CAD build for the part. Positions are in the model's coordinates, mm. A direction names the side the tool comes from. Give positions to 0.01 mm unless a question says otherwise; leave off trailing zeros. Write each loop counter-clockwise with the first axis right and the second up, starting at its lowest first coordinate (ties: lowest second). Pieces come first, ordered by that corner, then holes. Notation, with made-up numbers: (88.5, -23.75) -> (119.5, -23.75) arc R31 cw to (119.5, 13.25) -> close; hole circle Ø11 at (-16, -12). An arc over 180 degrees is marked (long way). Answer as a JSON object with one key per item and string values.
```python
from build123d import *

# Parameters (mm, degrees)
F0_R     = 9.525
F0_R_2   = 12.7
F1_DEPTH = 19.05
F2_R     = 34.925
F2_R_2   = 12.7
F3_DEPTH = 19.05
F4_R     = 34.925
F4_R_2   = 25.4
F5_DEPTH = 12.7
F7_DEPTH = 12.7


with BuildPart() as f1:
    # F0 (on Front) → F1 (new body)
    with BuildSketch(Plane.XZ):
        with BuildLine():
            Line((-60.325, -16.497784), (-22.225, -38.494829))
            ThreePointArc((-22.225, -38.494829), (-0.877898, -44.44133), (20.687394, -39.342524))
            Line((20.687394, -39.342524), (60.483871, -18.416429))
            ThreePointArc((60.483871, -18.416429), (71.607263, 0), (60.483871, 18.416429))
            Line((60.483871, 18.416429), (20.687394, 39.342524))
            ThreePointArc((20.687394, 39.342524), (-0.877898, 44.44133), (-22.225, 38.494829))
            Line((-22.225, 38.494829), (-60.325, 16.497784))
            ThreePointArc((-60.325, 16.497784), (-69.85, 0), (-60.325, -16.497784))
        make_face()
        with Locations((-50.8, 0)):
            Circle(F0_R, mode=Mode.SUBTRACT)
        Circle(F0_R_2, mode=Mode.SUBTRACT)
        with Locations((50.8, 0)):
            Circle(F0_R, mode=Mode.SUBTRACT)
    extrude(amount=F1_DEPTH)

    # F2 (on face) → F3 (join)
    with BuildSketch(Plane.XZ.offset(19.05)):
        Circle(F2_R)
        Circle(F2_R_2, mode=Mode.SUBTRACT)
    extrude(amount=F3_DEPTH)

    # F4 (on face) → F5 (join)
    with BuildSketch(Plane.XZ.offset(38.1)):
        Circle(F4_R)
        Circle(F4_R_2, mode=Mode.SUBTRACT)
    extrude(amount=F5_DEPTH)

    # F6 (on face) → F7 (cut)
    with BuildSketch(Plane.XZ.offset(50.8)):
        with BuildLine():
            Line((-6.35, 34.342876), (-6.35, 24.593444))
            ThreePointArc((-6.35, 24.593444), (0, 25.4), (6.35, 24.593444))
            Line((6.35, 24.593444), (6.35, 34.342876))
            ThreePointArc((6.35, 34.342876), (0, 34.925), (-6.35, 34.342876))
        make_face()
        with BuildLine():
            Line((34.342876, 6.35), (24.593444, 6.35))
            ThreePointArc((24.593444, 6.35), (25.4, 0), (24.593444, -6.35))
            Line((24.593444, -6.35), (34.342876, -6.35))
            ThreePointArc((34.342876, -6.35), (34.925, 0), (34.342876, 6.35))
        make_face()
        with BuildLine():
            Line((6.35, -34.342876), (6.35, -24.593444))
            ThreePointArc((6.35, -24.593444), (0, -25.4), (-6.35, -24.593444))
            Line((-6.35, -24.593444), (-6.35, -34.342876))
            ThreePointArc((-6.35, -34.342876), (0, -34.925), (6.35, -34.342876))
        make_face()
        with BuildLine():
            Line((-34.342876, -6.35), (-24.593444, -6.35))
            ThreePointArc((-24.593444, -6.35), (-25.4, 0), (-24.593444, 6.35))
            Line((-24.593444, 6.35), (-34.342876, 6.35))
            ThreePointArc((-34.342876, 6.35), (-34.925, 0), (-34.342876, -6.35))
        make_face()
    extrude(amount=-F7_DEPTH, mode=Mode.SUBTRACT)


solid = f1.part
```
1) Mould opens along X. For faces 6 (the flat face through (30, -45, 6.35)), 7 (the cylindrical face through (71.605, -9.392, -0.317)), 8 (the flat face through (-6.35, -45, -29)) say: released by +X, released by -X, zero draft, split by the parting line, or undercut.
Model answer:
{"face 6": "zero draft", "face 7": "released by +X", "face 8": "undercut"}
2) Slice it at B-B (z = 0). List the corners of the cut face in (x, y) (3 decimals), then the cut area to 3 significant figures.
Model answer:
{"outline": "(-69.85, -19.05) -> (-60.325, -19.05) -> (-60.325, 0) -> (-69.85, 0) -> close; (-41.275, -19.05) -> (-34.925, -19.05) -> (-34.925, -38.1) -> (-12.7, -38.1) -> (-12.7, 0) -> (-41.275, 0) -> close; (12.7, -38.1) -> (34.925, -38.1) -> (34.925, -19.05) -> (41.275, -19.05) -> (41.275, 0) -> (12.7, 0) -> close; (60.325, -19.05) -> (71.607, -19.05) -> (71.607, 0) -> (60.325, 0) -> close", "area": "2,330 mm2"}
3) Pin check, flat tips, straight feed: pin 1 (10.5 mm diameter, centred on y = -47.5, z = 31.5, fed in from -X); pin 2 (5 mm diameter, centred on x = 30, y = -47.5, fed in from -Z); pin 3 (8 mm diameter, centred on x = -31.5, y = -47, fed in from +Z). Stop position of each tip, or through.
Model answer:
{"pin 1": "stops at x = -23.04", "pin 2": "stops at z = -21.53", "pin 3": "stops at z = 21.53"}
4) Wall check: probe 1 along X at (y, z) = (-3, 1.5); probe 2 along Z at (x, y) = (0, -17.5); probe 3 along Z at (x, y) = (0, -28) (3 decimals). Give the ranges that are in metal, low to high.
Model answer:
{"probe 1": "x = -69.79 to -60.21, -41.39 to -12.61, 12.61 to 41.39, 60.21 to 71.55", "probe 2": "z = -44.45 to -12.7, 12.7 to 44.45", "probe 3": "z = -34.925 to -12.7, 12.7 to 34.925"}
5) 3-axis set-ups, long thin cutter, end or side, ignore diameter. For faces 1 (the flat face through (-21, -50.8, 21)), 2 (the flat face through (15, -38.1, 0)), 3 (the flat face through (-41.542, -9.392, -27.342)), 4 (the flat face through (6.35, -45, 29)), 5 (the flat face through (-29, -45, 6.35)): which of +Z, -Z, +X, -X, +Y, -Y reach the whole face in a straight line?
Model answer:
{"face 1": "+Z, -Z, +X, -X, -Y", "face 2": "-Y", "face 3": "-Z, -X, +Y, -Y", "face 4": "+Z, -Z, -Y", "face 5": "+X, -X, -Y"}
6) Slice it at C-C (y = -17). List the corners of the cut face in (x, z) (3 decimals).
Model answer:
{"outline": "(-60.325, -16.498) -> (-22.225, -38.495) arc R44.45 ccw to (20.687, -39.343) -> (60.484, -18.416) arc R20.807 ccw to (60.484, 18.416) -> (20.687, 39.343) arc R44.45 ccw to (-22.225, 38.495) -> (-60.325, 16.498) arc R19.05 ccw to start; hole circle Ø19.05 at (-50.8, 0); hole circle Ø25.4 at (0, 0); hole circle Ø19.05 at (50.8, 0)"}
7) Slice it at A-A (x = 0). List the corners of the cut face in (y, z) (3 decimals), then the cut area to 3 significant figures.
Model answer:
{"outline": "(-38.1, -34.925) -> (-19.05, -34.925) -> (-19.05, -44.45) -> (0, -44.45) -> (0, -12.7) -> (-38.1, -12.7) -> close; (-38.1, 12.7) -> (0, 12.7) -> (0, 44.45) -> (-19.05, 44.45) -> (-19.05, 34.925) -> (-38.1, 34.925) -> close", "area": "2,060 mm2"}
8) Slice it at D-D (z = -29). List the corners of the cut face in (x, y).
Model answer:
{"outline": "(-38.67, -19.05) -> (-19.46, -19.05) -> (-19.46, -50.8) -> (-6.35, -50.8) -> (-6.35, -38.1) -> (6.35, -38.1) -> (6.35, -50.8) -> (19.46, -50.8) -> (19.46, -19.05) -> (40.36, -19.05) -> (40.36, 0) -> (-38.67, 0) -> close"}
